```python
from build123d import *

# Parameters (mm, degrees)
SKETCH1_W                = 5
SKETCH1_H                = 25
BOSS_EXTRUDE1_DEPTH      = 25
BOSS_EXTRUDE1_DEPTH_BACK = 15
CUT_EXTRUDE1_START       = -15.25
CUT_EXTRUDE1_DEPTH       = 29.5
SKETCH5_R                = 2.5
CUT_EXTRUDE4_DEPTH       = 38.5
CUT_EXTRUDE4_DEPTH_BACK  = 8
CUT_EXTRUDE5_DEPTH       = 5.5
SKETCH7_R                = 1.5
CUT_EXTRUDE6_DEPTH       = 45.5


with BuildPart() as part:
    # Sketch1 → Boss-Extrude1 (new body, two sides)
    with BuildSketch(Plane.XY) as boss_extrude1_sk:
        Polygon((23.61, -22.25), (48.86, -22.25), (48.86, 22.25), (0, 22.25), (0, 17.25), (23.61, 17.25), align=None)
        with Locations((33.11, -0.5)):
            Rectangle(SKETCH1_W, SKETCH1_H, mode=Mode.SUBTRACT)
    extrude(amount=BOSS_EXTRUDE1_DEPTH)
    extrude(boss_extrude1_sk.sketch, amount=-BOSS_EXTRUDE1_DEPTH_BACK)

    # Sketch2 → Cut-Extrude1 (cut)
    with BuildSketch(Plane(origin=(0, 0, 0), x_dir=(1, 0, 0), z_dir=(0, 1, 0)).offset(CUT_EXTRUDE1_START)):
        with BuildLine():
            Line((37.86, 12), (48.86, 12))
            Line((48.86, 12), (48.86, -12))
            Line((48.86, -12), (37.86, -12))
            ThreePointArc((37.86, -12), (25.86, 0), (37.86, 12))
        make_face()
    extrude(amount=CUT_EXTRUDE1_DEPTH, mode=Mode.SUBTRACT)

    # Sketch5 → Cut-Extrude4 (cut, two sides)
    with BuildSketch(Plane(origin=(0, -15.25, 0), x_dir=(1, 0, 0), z_dir=(0, 1, 0))) as cut_extrude4_sk:
        with Locations((37.86, 0)):
            Circle(SKETCH5_R)
    extrude(amount=CUT_EXTRUDE4_DEPTH, mode=Mode.SUBTRACT)
    extrude(cut_extrude4_sk.sketch, amount=-CUT_EXTRUDE4_DEPTH_BACK, mode=Mode.SUBTRACT)

    # Sketch6 → Cut-Extrude5 (cut)
    with BuildSketch(Plane(origin=(0, 22.25, 0), x_dir=(1, 0, 0), z_dir=(0, 1, 0))):
        Polygon((41.91, 2.33826859), (37.86, 4.67653718), (33.81, 2.33826859), (33.81, -2.33826859), (37.86, -4.67653718), (41.91, -2.33826859), align=None)
    extrude(amount=-CUT_EXTRUDE5_DEPTH, mode=Mode.SUBTRACT)

    # Sketch7 → Cut-Extrude6 (cut, through all)
    with BuildSketch(Plane(origin=(0, 22.25, 0), x_dir=(1, 0, 0), z_dir=(0, 1, 0))):
        with Locations((2.5, 3)):
            Circle(SKETCH7_R)
        with Locations((17.5, 3)):
            Circle(SKETCH7_R)
        with Locations((17.5, -13)):
            Circle(SKETCH7_R)
        with Locations((2.5, -13)):
            Circle(SKETCH7_R)
    extrude(amount=-CUT_EXTRUDE6_DEPTH, mode=Mode.SUBTRACT)


solid = part.part
```
Check sheet for the modelled part. Datum: model origin and axes. Units: mm. A direction names the side the tool comes from. Coordinates: 2 decimals unless noted, no trailing zeros. Loops run counter-clockwise (first coordinate to the right, second up) from the corner with the lowest first, then second, coordinate; pieces in that order, holes last.
1) Release check for a two-part mould opening along Z. For faces 5 (the face through (25.863, -0.707, 0.264)), 6 (the face through (30.61, -1, -12)), 7 (the face through (30, 0, 25)) record: released by +Z, released by -Z, zero draft, split by the parting line, or undercut.
2) Gauge pin test, flat ends, axial feed: pin 1 (10 mm diameter, centred on x = 16, y = -10.5, fed in from +Z); pin 2 (1 mm diameter, centred on y = 9.5, z = 20.5, fed in from -X). Record the tip position at first contact, or that the pin passes through.
3) Sectioned sample at D-D (x = 45). Record the boundary of the cut face in (y, z).
4) Access from +Z, -Z, +X, -X, +Y, -Y to the whole of each face (thin tool, end or side, straight path). Record for faces 1 (the face through (23.61, -2, 5)), 2 (the face through (35.807, 19.538, 3.491)), 3 (the face through (38, 14.25, -3)), 4 (the face through (33, -13, -13)).
5) Sectioned sample at A-A (z = 13). Record the boundary of the cut face in (x, y), and give its area (3 significant figures).
6) Material ranges on probe 1 along Z at (x, y) = (17.5, 21.2); probe 2 along X at (y, z) = (19, 13); probe 3 along Z at (x, y) = (37, 16), recorded low to high.
7) Sectioned sample at C-C (y = 0). Record the boundary of the cut face in (x, z).
8) Sectioned sample at B-B (x = 17.5). Record the boundary of the cut face in (y, z), and give its area (3 significant figures).
Check sheet entries:
1. face 5: undercut
1. face 6: zero draft
1. face 7: released by +Z
2. pin 1: passes through
2. pin 2: stops at x = 23.61
3. outline: (-22.25, -15) - (22.25, -15) - (22.25, 25) - (-22.25, 25) - close; hole (-15.25, -12) - (14.25, -12) - (14.25, 12) - (-15.25, 12) - close
4. face 1: +Z, -Z, -X, -Y
4. face 2: +Y
4. face 3: +X
4. face 4: +Z, -Z
5. outline: (0, 17.25) - (1, 17.25) - (1, 22.25) - (0, 22.25) - close; (4, 17.25) - (16, 17.25) - (16, 22.25) - (4, 22.25) - close; (19, 17.25) - (23.61, 17.25) - (23.61, -22.25) - (48.86, -22.25) - (48.86, 22.25) - (19, 22.25) - close; hole (30.61, -13) - (35.61, -13) - (35.61, 12) - (30.61, 12) - close
5. area: 1,090 mm2
6. probe 1: z = -15 to -4.5, -1.5 to 11.5, 14.5 to 25
6. probe 2: x = 0 to 1, 4 to 16, 19 to 48.86
6. probe 3: z = -15 to -2.35, 2.35 to 25
7. outline: (23.61, -15) - (30.61, -15) - (30.61, -9.56) arc R12 cw to (30.61, 9.56) - (30.61, 25) - (23.61, 25) - close; (35.61, -15) - (48.86, -15) - (48.86, -12) - (37.86, -12) arc R12 cw to (35.61, -11.79) - close; (35.61, 11.79) arc R12 cw to (37.86, 12) - (48.86, 12) - (48.86, 25) - (35.61, 25) - close
8. outline: (17.25, -15) - (22.25, -15) - (22.25, -4.5) - (17.25, -4.5) - close; (17.25, -1.5) - (22.25, -1.5) - (22.25, 11.5) - (17.25, 11.5) - close; (17.25, 14.5) - (22.25, 14.5) - (22.25, 25) - (17.25, 25) - close
8. area: 170 mm2
